CAD build for the part. Positions are in the model's coordinates, mm. Round coordinates to 2 decimals unless told otherwise and drop trailing zeros. Write each loop counter-clockwise with the first axis right and the second up, starting at its lowest first coordinate (ties: lowest second). Pieces come first, ordered by that corner, then holes. Notation, with made-up numbers: (21.5, 19.5) - (42.5, 19.5) arc R31 ccw to (42.5, 49.5) - close; hole circle Ø9 at (-28.5, 15). An arc over 180 degrees is marked (long way). Answer in a Markdown table with one row per item.
```python
from build123d import *

# Parameters (mm, degrees)
F1_DEPTH = 17


with BuildPart() as f1:
    # F0 (on Top) → F1 (new body)
    with BuildSketch(Plane.XY):
        with BuildLine():
            ThreePointArc((-17.519922, -37.518273), (3.359597, -38.642575), (23.731816, -33.931834))
            ThreePointArc((23.731816, -33.931834), (35.145251, -16.411791), (41.251738, 3.586439))
            ThreePointArc((41.251738, 3.586439), (31.785653, 22.230784), (17.519922, 37.518273))
            ThreePointArc((17.519922, 37.518273), (-3.359597, 38.642575), (-23.731816, 33.931834))
            ThreePointArc((-23.731816, 33.931834), (-35.145251, 16.411791), (-41.251738, -3.586439))
            ThreePointArc((-41.251738, -3.586439), (-31.785653, -22.230784), (-17.519922, -37.518273))
        make_face()
    extrude(amount=-F1_DEPTH)


solid = f1.part
```
Q1. Drill centre lines: line 1 (Y direction, x = 11, z = -1); line 2 (X direction, y = 12.5, z = -13.5); line 3 (Y direction, x = -24, z = -15.25). Where is each one in solid material? Low to high.
Computed:
| item | result |
|---|---|
| line 1 | y = -37.58 to 38.5 |
| line 2 | x = -36.84 to 37.55 |
| line 3 | y = -31.62 to 33.62 |
Q2. Saw through at B-B on y = 26. List the corners of the cut face in (x, z).
Computed:
| item | result |
|---|---|
| outline | (-29.78, -17) - (28.97, -17) - (28.97, 0) - (-29.78, 0) - close |
Q3. Saw through at C-C on x = -26. List the corners of the cut face in (y, z), then the cut area to 3 significant figures.
Computed:
| item | result |
|---|---|
| outline | (-29.5, -17) - (31.21, -17) - (31.21, 0) - (-29.5, 0) - close |
| area | 1,030 mm2 |
Q4. Flat gauge pins, fed straight in: pin 1 (5 mm diameter, centred on y = 22, z = -4, fed in from -X); pin 2 (1.5 mm diameter, centred on y = 27, z = -12.5, fed in from -X); pin 3 (1.5 mm diameter, centred on x = 19.5, z = -11, fed in from +Y). Where does each tip first touch, or does it go through?
Computed:
| item | result |
|---|---|
| pin 1 | stops at x = -33.62 |
| pin 2 | stops at x = -29.61 |
| pin 3 | stops at y = 36.5 |
Q5. Saw through at A-A on z = -3.75. List the corners of the cut face in (x, y).
Computed:
| item | result |
|---|---|
| outline | (-41.25, -3.59) arc R74.65 ccw to (-17.52, -37.52) arc R74.65 ccw to (23.73, -33.93) arc R74.65 ccw to (41.25, 3.59) arc R74.65 ccw to (17.52, 37.52) arc R74.65 ccw to (-23.73, 33.93) arc R74.65 ccw to start |
